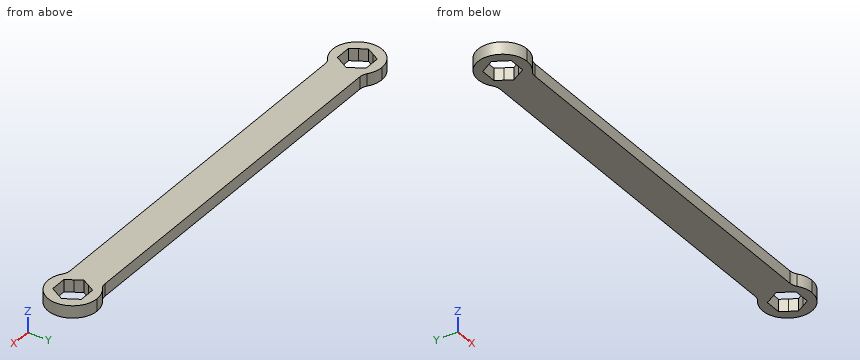
Autodesk Inventor part; units mm, degrees
ref_plane "YZ Plane" through (0, 0, 0) normal (1, 0, 0) x (0, 1, 0)
ref_plane "XZ Plane" through (0, 0, 0) normal (0, 1, 0) x (-1, 0, 0)
ref_plane "XY Plane" through (0, 0, 0) normal (0, 0, 1) x (1, 0, 0)
sketch "Sketch1" plane through (0, 0, 0) normal (0, 0, 1) x (1, 0, 0)
  circle A0 centre (-51.129, 0.0665) radius 3.5
  circle A1 centre (50.996, 0.0665) radius 3.5
  arc A2 (-51.129, 6.0665) -> (-51.129, -5.9335) centre (-51.129, 0.0665) ccw
  arc A3 (50.996, -5.9335) -> (50.996, 6.0665) centre (50.996, 0.0665) ccw
  arc A4 (-51.129, -5.9335) -> (-47.5672, -4.7619) centre (-51.129, 0.0665) ccw
  line L0 (-51.129, 0.0665) -> (-46.8864, -4.1761) construction
  line L1 (-51.129, 0.0665) -> (-51.129, -5.9335) construction
  arc A5 (-47.5672, 4.895) -> (-51.129, 6.0665) centre (-51.129, 0.0665) ccw
  line L2 (-51.129, 0.0665) -> (-46.8864, 4.3092) construction
  line L3 (-51.129, 0.0665) -> (-51.129, 6.0665) construction
  arc A6 (50.996, 6.0665) -> (47.4342, 4.895) centre (50.996, 0.0665) ccw
  line L4 (50.996, 0.0665) -> (46.7533, 4.3092) construction
  line L5 (50.996, 0.0665) -> (50.996, 6.0665) construction
  arc A7 (47.4342, -4.7619) -> (50.996, -5.9335) centre (50.996, 0.0665) ccw
  line L6 (50.996, 0.0665) -> (46.7533, -4.1761) construction
  line L7 (50.996, 0.0665) -> (50.996, -5.9335) construction
  line L8 (-45.7864, 4.3092) -> (45.6533, 4.3092)
  line L9 (-45.7864, -4.1761) -> (45.6533, -4.1761)
  arc A8 (-47.5672, 4.895) -> (-45.7864, 4.3092) centre (-45.7864, 7.3092) ccw
  arc A9 (-45.7864, -4.1761) -> (-47.5672, -4.7619) centre (-45.7864, -7.1761) ccw
  arc A10 (45.6533, 4.3092) -> (47.4342, 4.895) centre (45.6533, 7.3092) ccw
  arc A11 (47.4342, -4.7619) -> (45.6533, -4.1761) centre (45.6533, -7.1761) ccw
  line L10 (-47.0876, 0.0665) -> (-49.1083, -3.4335)
  line L11 (-49.1083, -3.4335) -> (-53.1498, -3.4335)
  line L12 (-53.1498, -3.4335) -> (-55.1705, 0.0665)
  line L13 (-55.1705, 0.0665) -> (-53.1498, 3.5665)
  line L14 (-53.1498, 3.5665) -> (-49.1083, 3.5665)
  line L15 (-49.1083, 3.5665) -> (-47.0876, 0.0665)
  line L16 (55.0374, 0.0665) -> (53.0167, -3.4335)
  line L17 (53.0167, -3.4335) -> (48.9752, -3.4335)
  line L18 (48.9752, -3.4335) -> (46.9545, 0.0665)
  line L19 (46.9545, 0.0665) -> (48.9752, 3.5665)
  line L20 (48.9752, 3.5665) -> (53.0167, 3.5665)
  line L21 (53.0167, 3.5665) -> (55.0374, 0.0665)
  point P0 (0, 0)
  point P1 (46.7533, 4.3092)
  dimension "d0" = 7
  dimension "d1" = 7
  dimension "d2" = 102.125
  dimension "d3" = 6
  dimension "d4" = 6
  dimension "d5" = 45
  dimension "d6" = 45
  dimension "d7" = 45
  dimension "d8" = 45
  dimension "d9" = 3
extrude "Extrusion2" add sketch "Sketch1" along normal blind 3
properties part number "2P.03.01.17.ZW.AileronCoupler"
Verification items for the finished model (mm, model axes). Coordinates: 2 decimals unless noted, no trailing zeros. Loops run counter-clockwise (first coordinate to the right, second up) from the corner with the lowest first, then second, coordinate; pieces in that order, holes last. Notation, with made-up numbers: (-20.5, 45) - (-5.5, 45) arc R21 ccw to (-5.5, 60) - close; hole circle Ø7 at (-22, 83). An arc over 180 degrees is marked (long way). Answer as a JSON object with one key per item and string values.
(1) Cross-section at C-C, the plane x = -14. Record the boundary of the cut face in (y, z).
Response:
{"outline": "(-4.18, 0) - (4.31, 0) - (4.31, 3) - (-4.18, 3) - close"}
(2) Go/stop test with flat-tipped pins: pin 1 Ø1.5 at (y, z) = (-3, 1.5) entering from +X; pin 2 Ø1.5 at (x, z) = (5.5, 1.5) entering from +Y. Record where each tip stops, or that it passes through.
Response:
{"pin 1": "stops at x = 56.53", "pin 2": "stops at y = 4.31"}
(3) Cross-section at A-A, the plane z = 2.25. Record the boundary of the cut face in (x, y) (1 decimal), then the cut area to 3 significant figures.
Response:
{"outline": "(-51.1, -5.9) arc R6 ccw to (-47.6, -4.8) arc R3 cw to (-45.8, -4.2) - (45.7, -4.2) arc R3 cw to (47.4, -4.8) arc R6 ccw to (51, -5.9) arc R6 ccw to (51, 6.1) arc R6 ccw to (47.4, 4.9) arc R3 cw to (45.7, 4.3) - (-45.8, 4.3) arc R3 cw to (-47.6, 4.9) arc R6 ccw to (-51.1, 6.1) arc R6 ccw to start; hole (-55.2, 0.1) - (-53.1, -3.4) - (-49.1, -3.4) - (-47.1, 0.1) - (-49.1, 3.6) - (-53.1, 3.6) - close; hole (47, 0.1) - (49, -3.4) - (53, -3.4) - (55, 0.1) - (53, 3.6) - (49, 3.6) - close", "area": "916 mm²"}
(4) Cross-section at B-B, the plane x = 50. Record the boundary of the cut face in (y, z), then the cut area to 3 significant figures.
Response:
{"outline": "(-5.85, 0) - (-3.43, 0) - (-3.43, 3) - (-5.85, 3) - close; (3.57, 0) - (5.98, 0) - (5.98, 3) - (3.57, 3) - close", "area": "14.5 mm²"}
(5) Scan lines: line 1 along X through (y, z) = (0.5, 0.4); line 2 along X through (y, z) = (-3, 0.2); line 3 along Y through (x, z) = (-2.5, 2.85). Record each from-to range of solid material in increasing order.
Response:
{"line 1": "x = -57.11 to -54.92, -47.34 to 47.2, 54.79 to 56.98", "line 2": "x = -56.29 to -53.4, -48.86 to 48.72, 53.27 to 56.15", "line 3": "y = -4.18 to 4.31"}
